Build history of the part. All positions in model axes, mm. A direction names the side the tool comes from. Give positions to 0.01 mm unless a question says otherwise; leave off trailing zeros. Write each loop counter-clockwise with the first axis right and the second up, starting at its lowest first coordinate (ties: lowest second). Pieces come first, ordered by that corner, then holes. Notation, with made-up numbers: (25, -21) -> (68, -21) arc R28 cw to (68, 5) -> close; hole circle Ø5 at (62, 71.5). An arc over 180 degrees is marked (long way). Write item = value, one per line. Start each with the question number.
Q1. Wall check: line 1 (X direction, y = 1.5, z = 25); line 2 (Z direction, x = -29, y = 5.5); line 3 (X direction, y = 9.5, z = -7.5). Give the ranges that are in metal, low to high.
Q2. Drop flat-ended pins along their axis: P1, Ø2, axis at x = -0.5, z = 15.5, coming from the -Y side; P2, Ø8, axis at x = 4, z = 23.5, coming from the -Y side; P3, Ø6, axis at x = 8.64, z = 27.89, coming from the +Y side; P4, Ø10, axis at x = 31.5, z = -35, coming from the -Y side. Give the stop position or say it passes through.
Q3. Saw through at B-B, the plane z = -6. List the corners of the cut face in (x, y), then the cut area to 3 significant figures.
Q4. Tool access for faces 3 (the face through (0, 4, -43)), 4 (the face through (-32, 9, 0)): list every direction of +Z, -Z, +X, -X, +Y, -Y with a clear straight run to the whole face (end or side of a thin tool).
Q5. Mould opens along Z. For faces 1 (the face through (41.99, 2.46, -42.15)), 2 (the face through (8.34, 9.014, 25.627)) say: pulls with the +Z half, pulls with the -Z half, needs draft (parallel to the pull), parting line crosses it, or undercut.
Q6. Saw through at A-A, the plane y = 2.25. List the corners of the cut face in (x, z).
Autodesk Inventor part; units mm, degrees
ref_plane "YZ Plane" through (0, 0, 0) normal (1, 0, 0) x (0, 1, 0)
ref_plane "XZ Plane" through (0, 0, 0) normal (0, 1, 0) x (-1, 0, 0)
sketch "Sketch1" plane through (0, 0, 0) normal (0, 1, 0) x (-1, 0, 0)
  line L0 (45, 35) -> (45, -35)
  line L1 (35, -45) -> (-35, -45)
  line L2 (-45, -35) -> (-45, 35)
  line L3 (-35, 45) -> (35, 45)
  line L4 (45, 45) -> (-45, -45) construction
  line L5 (45, -45) -> (-45, 45) construction
  arc A0 (35, -45) -> (45, -35) centre (35, -35) ccw
  arc A1 (-45, -35) -> (-35, -45) centre (-35, -35) ccw
  arc A2 (-35, 45) -> (-45, 35) centre (-35, 35) ccw
  arc A3 (45, 35) -> (35, 45) centre (35, 35) ccw
  point P0 (0, 0)
  dimension "d0" = 90
  dimension "d1" = 90
  dimension "d10" = 10
extrude "Extrusion1" add sketch "Sketch1" along normal blind 10
shell "Shell2" thickness 2 removed faces 1 at (-11.6667, 0, -15)
fillet "Fillet1" radius 5 1 edges at (-45, 10, 0)
sketch "Sketch2" plane through (0, 10, 0) normal (0, 1, 0) x (1, 0, 0)
  circle A0 centre (24.0106, 0) radius 10
  line L0 (-11.5, 11.5) -> (11.5, 11.5)
  line L1 (-11.5, -11.5) -> (-11.5, 11.5)
  line L2 (11.5, -11.5) -> (-11.5, -11.5)
  line L3 (11.5, 11.5) -> (11.5, -11.5)
  line L4 (-31.5, -10) -> (-16.5, -10)
  line L5 (-16.5, -10) -> (-16.5, 10)
  line L6 (-16.5, 10) -> (-31.5, 10)
  line L7 (-31.5, 10) -> (-31.5, -10)
  line L8 (-11.5, 22) -> (11.5, 22)
  line L9 (11.5, 22) -> (11.5, 28)
  line L10 (11.5, 28) -> (-11.5, 28)
  line L11 (-11.5, 28) -> (-11.5, 22)
  line L12 (12, 21.5) -> (-12, 21.5)
  line L13 (-12, 21.5) -> (-12, 28.5)
  line L14 (-12, 28.5) -> (12, 28.5)
  line L15 (12, 28.5) -> (12, 21.5)
  circle A1 centre (24.0106, 0) radius 10.5
  line L16 (12, 12) -> (-12, 12)
  line L17 (-12, 12) -> (-12, -12)
  line L18 (-12, -12) -> (12, -12)
  line L19 (12, -12) -> (12, 12)
  line L20 (-16, 10.5) -> (-16, -10.5)
  line L21 (-16, -10.5) -> (-32, -10.5)
  line L22 (-32, -10.5) -> (-32, 10.5)
  line L23 (-32, 10.5) -> (-16, 10.5)
  point P0 (0, 0)
  dimension "d13" = 0.5
  dimension "d14" = 0.5
  dimension "d15" = 0.5
  dimension "d16" = 0.5
extrude "Extrusion2" cut sketch "Sketch2" along normal through all both and the other way through all contours A0 | L0 L3 L2 L1 | L7 L6 L5 L4 | L11 L10 L9 L8 | L12 L13 L14 L15 | A1 | L19 L18 L17 L16 | L20 L21 L22 L23
sketch "Sketch3" plane through (-35, 8, -43) normal (0, -1, 0) x (1, 0, 0)
  circle A0 centre (35, 28.5) radius 1
  circle A1 centre (35, 57.5) radius 1
  circle A2 centre (51.5106, 33) radius 1.5
  circle A3 centre (66.5106, 33) radius 1.5
  circle A4 centre (51.5106, 60.4954) radius 1.5
  circle A5 centre (66.5106, 60.5) radius 1.5
  circle A6 centre (11, 31) radius 1.5
  arc A7 (37, 28.5) -> (33, 28.5) centre (35, 28.5) ccw
  circle A8 centre (35, 57.5) radius 2
  circle A9 centre (51.5106, 33) radius 2
  circle A10 centre (51.5106, 60.4954) radius 2
  circle A11 centre (66.5106, 60.5) radius 2
  circle A12 centre (66.5106, 33) radius 2
  circle A13 centre (11, 31) radius 1.35
  arc A14 (33, 26) -> (37, 26) centre (35, 26) ccw
  line L0 (53.5, 23) -> (15.5, 23)
  line L1 (33, 28.5) -> (33, 26)
  line L2 (37, 28.5) -> (37, 26)
  point P0 (35, 43)
  dimension "d19" = 4
  dimension "d20" = 4
  dimension "d21" = 4
  dimension "d22" = 2.7
  dimension "d32" = 3
extrude "Extrusion3" add sketch "Sketch3" along normal blind 1.4986 contours A0 | A1 | L2 A14 L1 A7 | A8
sketch "Sketch4" plane through (-35, 8, -43) normal (0, -1, 0) x (1, 0, 0)
  circle A0 centre (51.5106, 60.4954) radius 2
  circle A1 centre (66.5106, 60.5) radius 2
  circle A2 centre (66.5106, 33) radius 2
  circle A3 centre (51.5106, 33) radius 2
  point P0 (35, 43)
extrude "Extrusion4" add sketch "Sketch4" along normal blind 0.9906
sketch "Sketch5" plane through (-35, 8, -43) normal (0, -1, 0) x (1, 0, 0)
  circle A0 centre (11, 31) radius 1.35
  point P0 (35, 43)
extrude "Extrusion5" add sketch "Sketch5" along normal blind 2.4892
sketch "Sketch6" plane through (-35, 8, -43) normal (0, -1, 0) x (1, 0, 0)
  circle A0 centre (35, 8) radius 2
  circle A1 centre (35, 28.5) radius 2
  line L0 (15.5, 11) -> (53.5, 11)
  point P0 (35, 43)
  dimension "d29" = 3
extrude "Extrusion6" add sketch "Sketch6" along normal blind 1.4986 contours A0
sketch "Sketch7" plane through (31.5106, 7.0094, 17.5) normal (0, -1, 0) x (1, 0, 0)
  circle A0 centre (0, 0) radius 2
  circle A1 centre (-15, -0.0046) radius 2
  circle A2 centre (-31.5106, -3) radius 2
  circle A3 centre (-31.5106, -52.5) radius 2
  circle A4 centre (-55.5106, -29.5) radius 1.35
  line L0 (3.4894, -60.5) -> (-66.5106, -60.5)
  arc A5 (3.4894, -60.5) -> (11.4894, -52.5) centre (3.4894, -52.5) ccw
  line L1 (11.4894, 17.5) -> (11.4894, -52.5)
  arc A6 (11.4894, 17.5) -> (3.4894, 25.5) centre (3.4894, 17.5) ccw
  line L2 (-66.5106, 25.5) -> (3.4894, 25.5)
  arc A7 (-66.5106, 25.5) -> (-74.5106, 17.5) centre (-66.5106, 17.5) ccw
  line L3 (-74.5106, -52.5) -> (-74.5106, 17.5)
  arc A8 (-74.5106, -52.5) -> (-66.5106, -60.5) centre (-66.5106, -52.5) ccw
  line L4 (-19.5106, -5.5) -> (-19.5106, -29.5)
  line L5 (-19.5106, -29.5) -> (-43.5106, -29.5)
  line L6 (-43.5106, -29.5) -> (-43.5106, -5.5)
  line L7 (-43.5106, -5.5) -> (-19.5106, -5.5)
  line L8 (-63.5106, -7) -> (-47.5106, -7)
  line L9 (-47.5106, -7) -> (-47.5106, -28)
  line L10 (-47.5106, -28) -> (-63.5106, -28)
  line L11 (-63.5106, -28) -> (-63.5106, -7)
  line L12 (-43.5106, -46) -> (-43.5106, -39)
  line L13 (-43.5106, -39) -> (-19.5106, -39)
  line L14 (-19.5106, -39) -> (-19.5106, -46)
  line L15 (-19.5106, -46) -> (-43.5106, -46)
  arc A9 (-1.2, -25.9) -> (-13.8, -25.9) centre (-7.5, -17.5) ccw
  circle A10 centre (0, -27.5) radius 2
  arc A11 (-13.8, -25.9) -> (-1.2, -25.9) centre (-7.5, -17.5) ccw
  circle A12 centre (-15, -27.5) radius 2
  circle A13 centre (-31.5106, -3) radius 2
  arc A14 (-29.5106, -32) -> (-33.5106, -32) centre (-31.5106, -32) ccw
  line L16 (-29.5106, -32) -> (-29.5106, -34.5)
  arc A15 (-33.5106, -34.5) -> (-29.5106, -34.5) centre (-31.5106, -34.5) ccw
  line L17 (-33.5106, -34.5) -> (-33.5106, -32)
  circle A16 centre (0, 0) radius 2
  circle A17 centre (-15, -0.0046) radius 2
  circle A18 centre (0, 0) radius 0.75
  circle A19 centre (-15, -0.0046) radius 2
  circle A20 centre (-15, -0.0046) radius 0.75
  circle A21 centre (-31.5106, -3) radius 2
  circle A22 centre (-31.5106, -3) radius 0.75
  circle A23 centre (-15, -27.5) radius 2
  circle A24 centre (-15, -27.5) radius 0.75
  arc A25 (-29.5106, -32) -> (-33.5106, -32) centre (-31.5106, -32) ccw
  circle A26 centre (-31.5106, -32) radius 0.75
  circle A27 centre (0, -27.5) radius 0.75
  circle A28 centre (-31.5106, -35) radius 0.75
  circle A29 centre (-55.5106, -29.5) radius 0.5
  circle A30 centre (-31.5106, -52.5) radius 0.75
  point P0 (-31.5106, -17.5)
  dimension "d33" = 0.5
  dimension "d34" = 1.5
  dimension "d35" = 1
extrude "Extrusion7" cut sketch "Sketch7" along normal mid plane 4 contours A18 | A20 | A22 | A24 | A26 | A27 | A28 | A29 | A30
sketch "Sketch8" plane through (0, 0, 0) normal (0, -1, 0) x (1, 0, 0)
  arc A0 (35, -43) -> (43, -35) centre (35, -35) ccw
  line L0 (35, -43) -> (-35, -43)
  arc A1 (-43, -35) -> (-35, -43) centre (-35, -35) ccw
  line L1 (-43, -35) -> (-43, 35)
  arc A2 (-35, 43) -> (-43, 35) centre (-35, 35) ccw
  line L2 (-35, 43) -> (35, 43)
  arc A3 (43, 35) -> (35, 43) centre (35, 35) ccw
  line L3 (43, 35) -> (43, -35)
  line L4 (-35, -45) -> (35, -45)
  arc A4 (35, -45) -> (45, -35) centre (35, -35) ccw
  line L5 (45, -35) -> (45, 35)
  arc A5 (45, 35) -> (35, 45) centre (35, 35) ccw
  line L6 (35, 45) -> (-35, 45)
  arc A6 (-35, 45) -> (-45, 35) centre (-35, 35) ccw
  line L7 (-45, 35) -> (-45, -35)
  arc A7 (-45, -35) -> (-35, -45) centre (-35, -35) ccw
  circle A8 centre (0, 0) radius 39.5
  dimension "d38" = 79
sketch "Sketch9" plane through (0, 10, 0) normal (0, 1, 0) x (1, 0, 0)
  circle A0 centre (-19.6342, -26.7992) radius 1.778
  circle A1 centre (-9.2112, -27.769) radius 1.778
  circle A2 centre (-0.509, -33.4037) radius 1.778
  circle A3 centre (-0.4072, -26.2997) radius 1.778
  circle A4 centre (8.6368, -27.8855) radius 1.778
  circle A5 centre (17.3608, -26.6743) radius 1.778
  circle A6 centre (-19.6342, -26.7992) radius 2.278
  circle A7 centre (-9.2112, -27.769) radius 2.278
  circle A8 centre (-0.4072, -26.2997) radius 2.278
  circle A9 centre (-0.509, -33.4037) radius 2.278
  circle A10 centre (8.6368, -27.8855) radius 2.278
  circle A11 centre (17.3608, -26.6743) radius 2.278
  point P0 (0, 0)
  dimension "d39" = 0.5
extrude "Extrusion8" cut sketch "Sketch9" along normal through all both and the other way through all contours A0 | A1 | A2 | A3 | A4 | A5 | A6 | A7 | A8 | A9 | A10 | A11
sketch "Sketch10" plane through (-35, 8, -43) normal (0, -1, 0) x (1, 0, 0)
  circle A0 centre (8.9998, 68.5014) radius 1.5 construction
  circle A1 centre (27, 78.0009) radius 1.5 construction
  circle A2 centre (26.9997, 64.0009) radius 1.5 construction
  circle A3 centre (43, 78.0005) radius 1.5 construction
  circle A4 centre (42.9997, 64.0005) radius 1.5 construction
  circle A5 centre (60.9998, 68.5001) radius 1.5 construction
  circle A6 centre (8.9998, 68.5014) radius 2
  circle A7 centre (27, 78.0009) radius 2
  circle A8 centre (26.9997, 64.0009) radius 2
  circle A9 centre (42.9997, 64.0005) radius 2
  circle A10 centre (43, 78.0005) radius 2
  circle A11 centre (60.9998, 68.5001) radius 2
  circle A12 centre (8.9998, 68.5014) radius 0.75
  circle A13 centre (27, 78.0009) radius 0.75
  circle A14 centre (26.9997, 64.0009) radius 0.75
  circle A15 centre (43, 78.0005) radius 0.75
  circle A16 centre (42.9997, 64.0005) radius 0.75
  circle A17 centre (60.9998, 68.5001) radius 0.75
  point P0 (35, 43)
  dimension "d42" = 4
  dimension "d43" = 1.5
extrude "Extrusion9" add sketch "Sketch10" along normal blind 3
equation "\"d13\" = d14"
equation "\"d15\" = d14"
equation "\"d16\" = d14"
properties material "LCP Plastic"
Report:
q1.line_1 = -45 to -43, 43 to 45
q1.line_2 = -44.97 to -43, 43 to 44.97
q1.line_3 = -42.18 to -32, -16 to -12, 12 to 16.66, 31.36 to 42.18
q2.P1 = 6.5
q2.P2 = 5
q2.P3 = 10
q2.P4 = 8
q3.outline = (-45, 0) -> (-43, 0) -> (-43, 8) -> (-32, 8) -> (-32, 10) -> (-40, 10) arc R5 ccw to (-45, 5) -> close; (-16, 8) -> (-12, 8) -> (-12, 10) -> (-16, 10) -> close; (12, 8) -> (15.39, 8) -> (15.39, 10) -> (12, 10) -> close; (32.63, 8) -> (43, 8) -> (43, 0) -> (45, 0) -> (45, 5) arc R5 ccw to (40, 10) -> (32.63, 10) -> close
q3.area = 86.8 mm2
q4.face_3 = -Y
q4.face_4 = +Y, -Y
q5.face_1 = pulls with the -Z half
q5.face_2 = undercut
q6.outline = (-45, -35) arc R10 ccw to (-35, -45) -> (35, -45) arc R10 ccw to (45, -35) -> (45, 35) arc R10 ccw to (35, 45) -> (-35, 45) arc R10 ccw to (-45, 35) -> close; hole (-43, -35) arc R8 ccw to (-35, -43) -> (35, -43) arc R8 ccw to (43, -35) -> (43, 35) arc R8 ccw to (35, 43) -> (-35, 43) arc R8 ccw to (-43, 35) -> close
